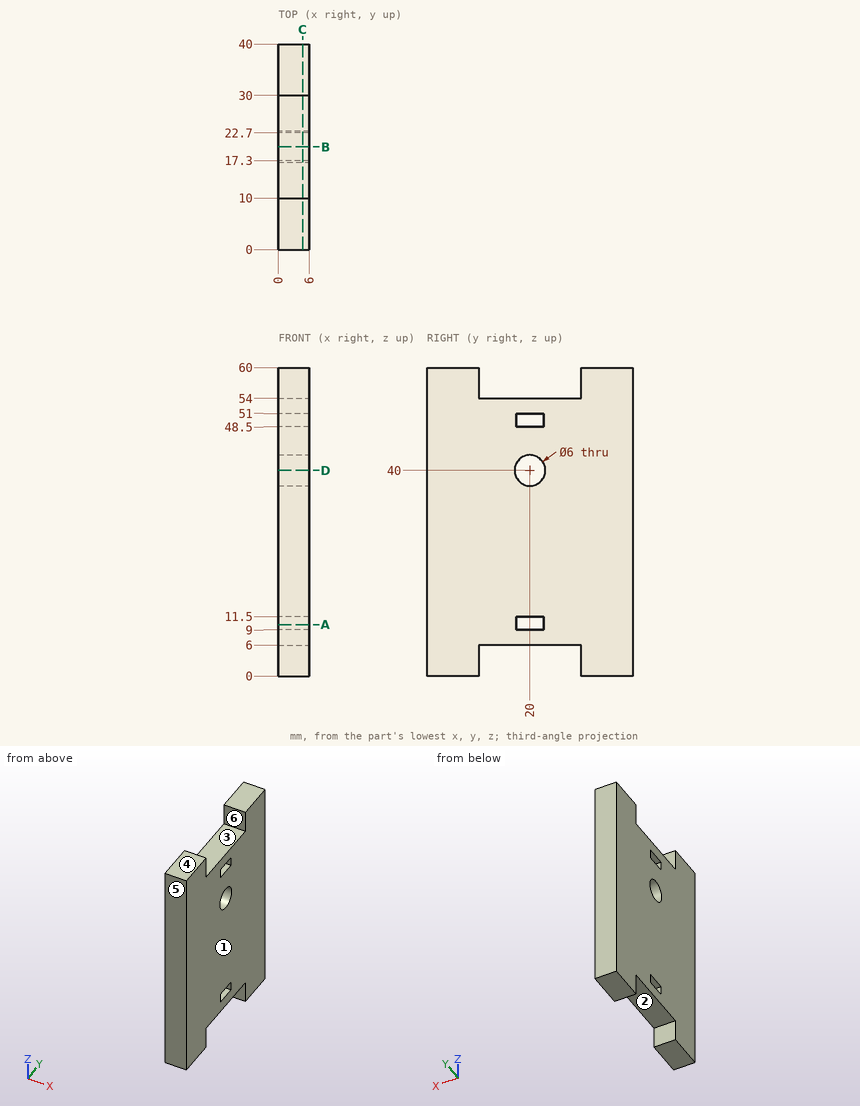
Geometry check sheet. Reference: drawing and pictorial views, mm from the part's lowest x, y, z. A direction names the side the tool comes from. Round coordinates to 2 decimals unless told otherwise and drop trailing zeros. Order: outer loops, then holes, each group sorted by start corner. A loop starts at its lowest first (then second) coordinate and runs counter-clockwise, first axis right, second up. Notation, with made-up numbers: (-38.5, 49) - (-18.5, 49) arc R25 ccw to (-18.5, 81) - close; hole circle Ø9 at (75.5, 61). An arc over 180 degrees is marked (long way). Use a Markdown table: item, result. Add a question column.
1) Mould release check, pull along Y, two halves, no side actions. Record for the marked faces 4, 5 and 6: released by +Y, released by -Y, zero draft, split by the parting line, or undercut.
2) Gauge pin test, flat ends, axial feed: P1, Ø1.6, axis at x = 2, y = 20.5, coming from the +Z side; P2, Ø2, axis at x = 1.5, z = 10, coming from the -Y side; P3, Ø1.6, axis at x = 3.5, y = 20, coming from the -Z side. Record the tip position at first contact, or that the pin passes through.
3) Section check C-C (x = 4.75). Record the cut outline in (y, z), then the cut area to 3 significant figures.
4) Section check B-B (y = 20). Record the cut outline in (x, z), then the cut area to 3 significant figures.
5) Section check D-D (z = 40). Record the cut outline in (x, y), then the cut area to 3 significant figures.
6) Section check A-A (z = 10). Record the cut outline in (x, y), then the cut area to 3 significant figures.
7) Thickness scan on line 1 along Z through (x, y) = (2.55, 20); line 2 along Y through (x, z) = (4.15, 57); line 3 along Z through (x, y) = (1.7, 16.5). Record the ranges inside material, lowest first.
8) Set-up check for the marked faces 1, 2 and 3: record each of +Z, -Z, +X, -X, +Y, -Y from which the full face is reachable in a straight line by a thin tool's end or side.
Established:
| question | item | result |
|---|---|---|
| 1 | face 4 | zero draft |
| 1 | face 5 | released by -Y |
| 1 | face 6 | undercut |
| 2 | P1 | z = 54 |
| 2 | P2 | y = 0 |
| 2 | P3 | z = 6 |
| 3 | outline | (0, 0) - (10, 0) - (10, 6) - (30, 6) - (30, 0) - (40, 0) - (40, 60) - (30, 60) - (30, 54) - (10, 54) - (10, 60) - (0, 60) - close; hole circle Ø6 at (20, 40); hole (17.3, 9) - (22.7, 9) - (22.7, 11.5) - (17.3, 11.5) - close; hole (17.3, 48.5) - (22.7, 48.5) - (22.7, 51) - (17.3, 51) - close |
| 3 | area | 2,100 mm2 |
| 4 | outline | (0, 6) - (6, 6) - (6, 9) - (0, 9) - close; (0, 11.5) - (6, 11.5) - (6, 37) - (0, 37) - close; (0, 43) - (6, 43) - (6, 48.5) - (0, 48.5) - close; (0, 51) - (6, 51) - (6, 54) - (0, 54) - close |
| 4 | area | 222 mm2 |
| 5 | outline | (0, 0) - (6, 0) - (6, 17) - (0, 17) - close; (0, 23) - (6, 23) - (6, 40) - (0, 40) - close |
| 5 | area | 204 mm2 |
| 6 | outline | (0, 0) - (6, 0) - (6, 17.3) - (0, 17.3) - close; (0, 22.7) - (6, 22.7) - (6, 40) - (0, 40) - close |
| 6 | area | 208 mm2 |
| 7 | line 1 | 6 to 9, 11.5 to 37, 43 to 48.5, 51 to 54 |
| 7 | line 2 | 0 to 10, 30 to 40 |
| 7 | line 3 | 6 to 54 |
| 8 | face 1 | +Z, -Z, +X, +Y, -Y |
| 8 | face 2 | -Z, +X, -X |
| 8 | face 3 | +Z, +X, -X |
